Autodesk Inventor part; units mm, degrees
ref_plane "YZ Plane" through (0, 0, 0) normal (1, 0, 0) x (0, 1, 0)
ref_plane "XZ Plane" through (0, 0, 0) normal (0, 1, 0) x (-1, 0, 0)
ref_plane "XY Plane" through (0, 0, 0) normal (0, 0, 1) x (1, 0, 0)
sketch "Sketch1" plane through (0, 0, 0) normal (0, 0, 1) x (1, 0, 0)
  line L0 (19.75, -5) -> (-19.75, -5)
  line L1 (-19.75, -5) -> (-19.75, 5)
  line L2 (-19.75, 5) -> (19.75, 5)
  line L3 (19.75, 5) -> (19.75, -5)
  line L4 (19.75, -5) -> (-19.75, 5) construction
  line L5 (-19.75, -5) -> (19.75, 5) construction
  line L6 (16, 0) -> (-16, 0) construction
  point P0 (0, 0)
  point P1 (0, 5)
  point P2 (0, 0)
  dimension "d0" = 39.5
  dimension "d1" = 10
  dimension "d6" = 32
extrude "Extrusion1" add sketch "Sketch1" along normal blind 1.8796
fillet "Fillet1" radius 2 4 edges at (-19.75, 5, 0.9398) (-19.75, -5, 0.9398) (19.75, -5, 0.9398) (19.75, 5, 0.9398)
hole "Hole1" at (16, 0, 0) at (-16, 0, 0) direction (0, 0, 1) diameter 2.459 end through all
properties part number "Cowling Magnetic Catch" material "Steel, Carbon"
Part model, mm, in its own coordinate system. Round coordinates to 2 decimals unless told otherwise and drop trailing zeros. Write each loop counter-clockwise with the first axis right and the second up, starting at its lowest first coordinate (ties: lowest second). Pieces come first, ordered by that corner, then holes. Notation, with made-up numbers: M 75,48 L 124,48 A16 ccw 124,74 Z; hole C 15.5,9 d7. An arc over 180 degrees is marked long. One line per question, with ' | ' between items.
(1) Saw through at D-D on y = 4.25. Write the cut outline in (x, z).
Answer key:
outline: M -19.31,0 L 19.31,0 L 19.31,1.88 L -19.31,1.88 Z
(2) Two-plate mould, pull along Y, no slides. Class faces 1 (the face through (-17.22, -0.16, 0.95)), 2 (the face through (19.15, -4.43, 0.95)), 3 (the face through (14.78, -0.16, 0.95)), 4 (the face through (-19.15, 4.43, 0.95)): released by +Y, released by -Y, zero draft, split by the parting line, or undercut.
Answer key:
face 1: undercut | face 2: released by -Y | face 3: undercut | face 4: released by +Y
(3) Probe line 1 along X through (y, z) = (0, 0.8); line 2 along Y through (x, z) = (-16, 1); line 3 along X through (y, z) = (3.5, 0.5). List the from-to ranges inside material, lowest first.
Answer key:
line 1: x = -19.75 to -17.23, -14.77 to 14.77, 17.23 to 19.75 | line 2: y = -5 to -1.23, 1.23 to 5 | line 3: x = -19.69 to 19.69
(4) Saw through at B-B on x = -16. Write the cut outline in (y, z), then the cut area to 3 significant figures.
Answer key:
outline: M -5,0 L -1.23,0 L -1.23,1.88 L -5,1.88 Z; M 1.23,0 L 5,0 L 5,1.88 L 1.23,1.88 Z | area: 14.2 mm^2
(5) Saw through at A-A on z = 1. Write the cut outline in (x, y).
Answer key:
outline: M -19.75,-3 A2 ccw -17.75,-5 L 17.75,-5 A2 ccw 19.75,-3 L 19.75,3 A2 ccw 17.75,5 L -17.75,5 A2 ccw -19.75,3 Z; hole C -16,0 d2.46; hole C 16,0 d2.46
(6) Pin check, flat tip, straight feed: pin 1 (2 mm diameter, centred on x = -16, y = 0, fed in from +Z). Stop position of the tip, or through.
Answer key:
pin 1: passes through
(7) Saw through at C-C on y = -0.5. Write the cut outline in (x, z), then the cut area to 3 significant figures.
Answer key:
outline: M -19.75,0 L -17.12,0 L -17.12,1.88 L -19.75,1.88 Z; M -14.88,0 L 14.88,0 L 14.88,1.88 L -14.88,1.88 Z; M 17.12,0 L 19.75,0 L 19.75,1.88 L 17.12,1.88 Z | area: 65.8 mm^2
